Model file for the job. Use its own axes, mm. Give positions to 0.01 mm unless a question says otherwise; leave off trailing zeros. Loops run counter-clockwise (first coordinate to the right, second up) from the corner with the lowest first, then second, coordinate; pieces in that order, holes last. Notation, with made-up numbers: (19, -30.5) - (44, -30.5) arc R28 ccw to (44, -11.5) - close; hole circle Ø1 at (13, -21). An arc over 180 degrees is marked (long way). Use a Markdown table: item, result.
from build123d import *

# Parameters (mm, degrees)
F0_W     = 100
F0_H     = 70
F1_DEPTH = 2.54
F2_W     = 94.92
F2_H     = 64.92
F2_W_2   = 92.38
F2_H_2   = 62.38
F3_DEPTH = 0.508
F4_W     = 8.86
F4_H     = 0.508
F5_DEPTH = 25.4


with BuildPart() as f1:
    # F0 (on Top) → F1 (new body)
    with BuildSketch(Plane.XY):
        Rectangle(F0_W, F0_H)
    extrude(amount=F1_DEPTH)

    # F2 (on face) → F3 (join)
    with BuildSketch(Plane.XY.offset(2.54)):
        Rectangle(F2_W, F2_H)
        Rectangle(F2_W_2, F2_H_2, mode=Mode.SUBTRACT)
    extrude(amount=F3_DEPTH)

    # F4 (on face) → F5 (cut)
    with BuildSketch(Plane.XZ.offset(32.46)):
        with Locations((0.07, 2.794)):
            Rectangle(F4_W, F4_H)
    extrude(amount=-F5_DEPTH, mode=Mode.SUBTRACT)


solid = f1.part
(1) Slice it at A-A, the plane x = 39.5. Write the cut outline in (y, z).
Computed:
| item | result |
|---|---|
| outline | (-35, 0) - (35, 0) - (35, 2.54) - (32.46, 2.54) - (32.46, 3.05) - (31.19, 3.05) - (31.19, 2.54) - (-31.19, 2.54) - (-31.19, 3.05) - (-32.46, 3.05) - (-32.46, 2.54) - (-35, 2.54) - close |
(2) Slice it at B-B, the plane y = 15. Write the cut outline in (x, z).
Computed:
| item | result |
|---|---|
| outline | (-50, 0) - (50, 0) - (50, 2.54) - (47.46, 2.54) - (47.46, 3.05) - (46.19, 3.05) - (46.19, 2.54) - (-46.19, 2.54) - (-46.19, 3.05) - (-47.46, 3.05) - (-47.46, 2.54) - (-50, 2.54) - close |
(3) Mould opens along X. For faces 1 (the flat face through (-0.2, 31.4, 3.048)), 2 (the flat face through (-1, 0, 2.54)), 3 (the flat face through (-50, 0, 1)), 4 (the flat face through (50, 0, 1)) say: pulls with the +X half, pulls with the -X half, needs draft (parallel to the pull), parting line crosses it, or undercut.
Computed:
| item | result |
|---|---|
| face 1 | needs draft |
| face 2 | undercut |
| face 3 | pulls with the -X half |
| face 4 | pulls with the +X half |
(4) Pin check, flat tips, straight feed: P1, Ø1.5, axis at x = 3.5, y = 20, coming from the +Z side; P2, Ø0.6, axis at x = 25, z = 3, coming from the +Y side; P3, Ø10, axis at x = 35.5, y = -9.5, coming from the -Z side; P4, Ø0.6, axis at x = 17.5, z = 3, coming from the -Y side. Stop position of each tip, or through.
Computed:
| item | result |
|---|---|
| P1 | z = 2.54 |
| P2 | y = 32.46 |
| P3 | z = 0 |
| P4 | y = -32.46 |
(5) Drill centre lines: probe 1 along Y at (x, z) = (16.5, 2.6); probe 2 along X at (y, z) = (-1.5, 2.65); probe 3 along Z at (x, y) = (-35.5, 3). Where is each one in solid material? Low to high. Write a range as [from, to].
Computed:
| item | result |
|---|---|
| probe 1 | [-32.46, -31.19], [31.19, 32.46] |
| probe 2 | [-47.46, -46.19], [46.19, 47.46] |
| probe 3 | [0, 2.54] |
